Verification items for this drawing (mm, ordinates from the low corner). Round coordinates to 2 decimals unless told otherwise and drop trailing zeros. Write each loop counter-clockwise with the first axis right and the second up, starting at its lowest first coordinate (ties: lowest second). Pieces come first, ordered by that corner, then holes. Notation, with made-up numbers: (-32, 56) -> (4, 56) arc R36 cw to (4, 95) -> close; hole circle Ø9 at (38.5, 42.25). An arc over 180 degrees is marked (long way). Use one line per item in the form item = value. Start each with the question number.
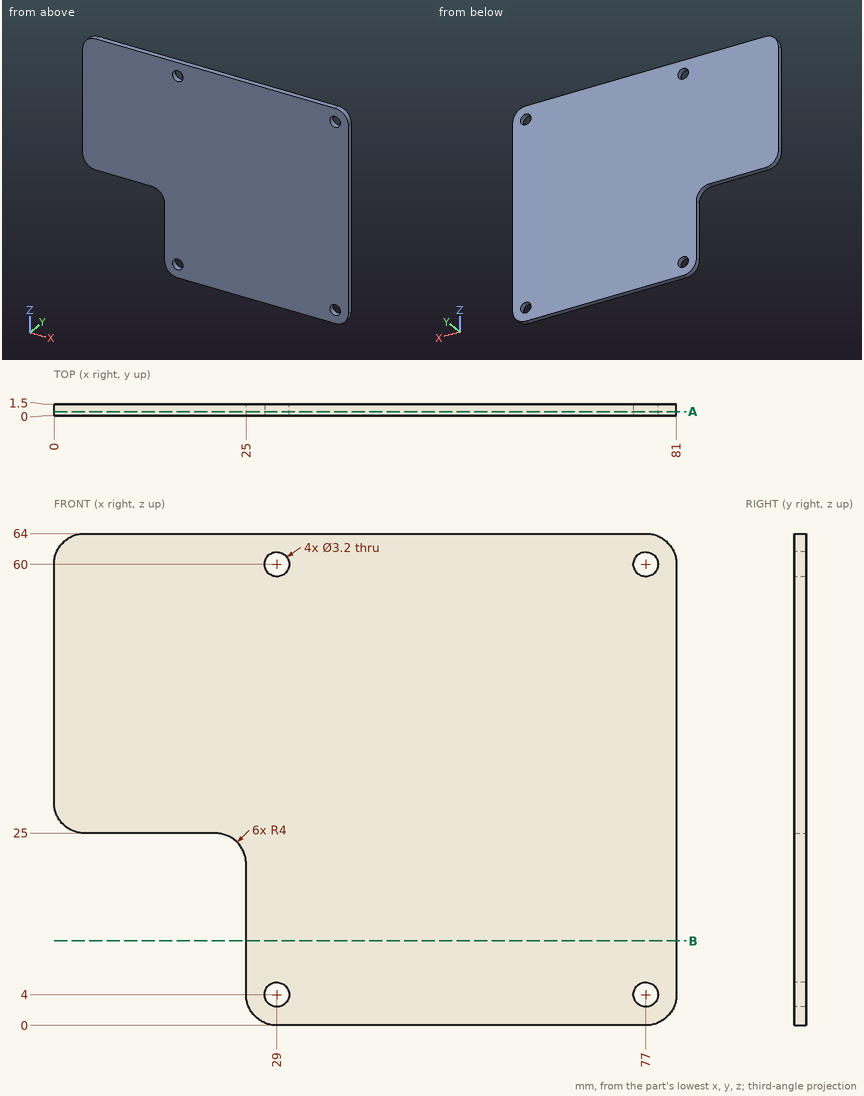
1. Depth check by flat-ended pin: pin 1 (0.8 mm diameter, centred on y = 0.5, z = 16, fed in from -X). Enter the tip coordinate at first touch or a pass-through.
2. Sectioned sample at B-B (z = 11). Enter the section's corners in (x, y).
3. Sectioned sample at A-A (y = 0.5). Enter the section's corners in (x, z).
4. Scan lines: probe 1 along X at (y, z) = (1.05, 60); probe 2 along Z at (x, y) = (77, 0.5); probe 3 along Z at (x, y) = (10, 0.25). Record each from-to range of solid material in increasing order.
Returned:
q1.pin_1 = 25
q2.outline = (25, 0) -> (81, 0) -> (81, 1.5) -> (25, 1.5) -> close
q3.outline = (0, 29) arc R4 ccw to (4, 25) -> (21, 25) arc R4 cw to (25, 21) -> (25, 4) arc R4 ccw to (29, 0) -> (77, 0) arc R4 ccw to (81, 4) -> (81, 60) arc R4 ccw to (77, 64) -> (4, 64) arc R4 ccw to (0, 60) -> close; hole circle Ø3.2 at (29, 4); hole circle Ø3.2 at (29, 60); hole circle Ø3.2 at (77, 4); hole circle Ø3.2 at (77, 60)
q4.probe_1 = 0 to 27.4, 30.6 to 75.4, 78.6 to 81
q4.probe_2 = 0 to 2.4, 5.6 to 58.4, 61.6 to 64
q4.probe_3 = 25 to 64
